Autodesk Fusion 360 part; units mm, degrees
sketch "Sketch1" plane through (0, 0, 0) normal (0, 1, 0) x (1, 0, 0)
  line L0 (0, 0) -> (65, 0)
  line L1 (65, 0) -> (65, 5)
  line L2 (65, 5) -> (80, 5)
  line L3 (80, 5) -> (80, -35)
  line L4 (80, -35) -> (0, -35)
  line L5 (0, -35) -> (-15, -35)
  line L6 (-15, -35) -> (-15, 5)
  line L7 (-15, 5) -> (0, 5)
  line L8 (0, 5) -> (0, 0)
  line L9 (32.5, 0) -> (32.5, -35) construction
  line L10 (32.5, 0) -> (4.5, 0) construction
  line L11 (32.5, 0) -> (60.5, 0) construction
  line L12 (60.5, 0) -> (60.5, -17) construction
  line L13 (56.5, -17) -> (8.5, -17)
  line L14 (4.5, -21) -> (4.5, -35)
  line L15 (60.5, -21) -> (60.5, -35)
  arc A0 (8.5, -17) -> (4.5, -21) centre (8.5, -21) ccw
  arc A1 (60.5, -21) -> (56.5, -17) centre (56.5, -21) ccw
  point P0 (4.5, -17)
  dimension "d1" = 65
  dimension "d2" = 28
  dimension "d3" = 28
  dimension "d4" = 17
  dimension "d5" = 56
  dimension "d6" = 4
  dimension "d7" = 4
extrude "Extrude1" add sketch "Sketch1" along normal blind 50 contours L0 L1 L2 L3 L4 L5 L6 L7 L8 L13 L14 L15 A0 A1
sketch "Sketch2" plane through (0, 0, 35) normal (0, 0, 1) x (1, 0, 0)
  line L0 (-15, 0) -> (4.5, 0)
  line L1 (4.5, 0) -> (4.5, 50)
  line L2 (4.5, 50) -> (-15, 50)
  line L3 (-15, 50) -> (-15, 0)
  line L4 (-15, 25) -> (80, 25) construction
  line L5 (32.5, 0.0866) -> (32.5, 50) construction
  line L6 (32.5, 25) -> (72.5, 25) construction
  line L7 (72.5, 25) -> (72.5, 41.75) construction
  line L8 (72.5, 25) -> (72.5, 8.25) construction
  line L9 (72.5, 41.75) -> (-7.5, 41.75) construction
  line L10 (72.5, 8.25) -> (-7.5, 8.25) construction
  point P0 (-7.5, 41.75)
  point P1 (72.5, 41.75)
  point P2 (72.5, 8.25)
  point P3 (-7.5, 8.25)
  dimension "d10" = 40
  dimension "d11" = 16.75
  dimension "d12" = 16.75
  dimension "d13" = 80
  dimension "d14" = 80
hole "Hole1" at (-7.5, 41.75, 35) at (72.5, 41.75, 35) at (72.5, 8.25, 35) at (-7.5, 8.25, 35) direction (0, 0, -1) diameter 5.5 depth 40 tip angle 118 counterbore diameter 9 counterbore depth 22
sketch "Sketch3" plane through (80, 0, 0) normal (1, 0, 0) x (0, 0, -1)
  line L0 (-35, 0) -> (5, 0)
  line L1 (5, 0) -> (5, 50)
  line L2 (5, 50) -> (-35, 50)
  line L3 (-35, 50) -> (-35, 0)
  line L4 (5, 25) -> (-35, 25) construction
  line L5 (-28.6189, 25) -> (-28.6189, 33) construction
  line L6 (-28.6189, 33) -> (-28.6189, 17) construction
  point P0 (-28.6189, 33)
  point P1 (-28.6189, 17)
hole "Hole2" at (80, 17, 28.6189) at (80, 33, 28.6189) direction (-1, 0, 0) diameter 3.2 depth 40 tip angle 118 counterbore diameter 7 counterbore depth 10
The model under review builds one solid part; all positions refer to its coordinate system, in mm. A direction names the side the tool comes from. Round coordinates to 2 decimals unless told otherwise and drop trailing zeros. Order: outer loops, then holes, each group sorted by start corner. A loop starts at its lowest first (then second) coordinate and runs counter-clockwise, first axis right, second up. Notation, with made-up numbers: (-21, 7) -> (14, 7) arc R20 ccw to (14, 22) -> close; hole circle Ø9 at (-11, 36). An arc over 180 degrees is marked (long way). One line per item, written item: value. Start each with the question number.
Q1. Clearance check with flat-ended pins moving along their axes: pin 1 Ø12 at (x, z) = (8.5, 21.5) entering from +Y; pin 2 Ø8 at (x, y) = (48.5, 25.5) entering from -Z; pin 3 Ø6 at (x, y) = (50, 28) entering from +Z; pin 4 Ø6.5 at (x, y) = (72.5, 8.25) entering from +Z. State where each tip first meets the part, or that it passes through.
Q2. Wall thickness on line 1 (Y direction, x = -7.5, z = 29.5); line 2 (X direction, y = 8, z = 7); line 3 (Z direction, x = 73, y = 17): over which ranges is each line inside the solid? List them lowest first.
Q3. Take a section at D-D (z = 7). Write out the cut boundary in (x, y).
Q4. Machinability: for faces 4 (the face through (70, 34, 27)), 5 (the face through (33, 25, 17)), 6 (the face through (-5, 25, 35)), 7 (the face through (65, 25, -2)), 8 (the face through (68.706, 39.331, 23.846)), which of the approach directions +Z, -Z, +X, -X, +Y, -Y give a long, thin tool a straight path to every point of the face, cutting with its end or side? Answer none if there is none.
Q5. Take a section at A-A (x = 72.5). Write out the cut boundary in (y, z), and give its area (3 significant figures).
Q6. Take a section at C-C (y = 17). Write out the cut boundary in (x, z).
Q7. Take a section at B-B (z = 23.5). Write out the cut boundary in (x, y).
Q8. Mouldability with a two-part tool opening along Y and no side actions: class faces 1 (the face through (32, 50, 15)), 2 (the face through (4.5, 25, 28)), 3 (the face through (-7.6, 44.5, 3.9)) as released by +Y, released by -Y, zero draft, split by the parting line, or undercut.
Reported:
1. pin 1: stops at y = 50
1. pin 2: stops at z = 0
1. pin 3: stops at z = 17
1. pin 4: stops at z = 13
2. line 1: y = 0 to 3.75, 12.75 to 37.25, 46.25 to 50
2. line 2: x = -15 to -10.24, -4.76 to 69.76, 75.24 to 80
2. line 3: z = -5 to 25.12, 32.12 to 35
3. outline: (-15, 0) -> (80, 0) -> (80, 50) -> (-15, 50) -> close; hole circle Ø5.5 at (-7.5, 8.25); hole circle Ø5.5 at (-7.5, 41.75); hole circle Ø5.5 at (72.5, 8.25); hole circle Ø5.5 at (72.5, 41.75)
4. face 4: +X
4. face 5: +Z, +Y, -Y
4. face 6: +Z, +X, -X, +Y, -Y
4. face 7: -Z, +Y, -Y
4. face 8: +Z
5. outline: (0, -5) -> (5.5, -5) -> (5.5, 13) -> (3.75, 13) -> (3.75, 35) -> (0, 35) -> close; (11, -5) -> (39, -5) -> (39, 13) -> (37.25, 13) -> (37.25, 35) -> (12.75, 35) -> (12.75, 13) -> (11, 13) -> close; (44.5, -5) -> (50, -5) -> (50, 35) -> (46.25, 35) -> (46.25, 13) -> (44.5, 13) -> close; hole circle Ø7 at (17, 28.62); hole circle Ø7 at (33, 28.62)
5. area: 1,330 mm2
6. outline: (-15, -5) -> (0, -5) -> (0, 0) -> (65, 0) -> (65, -5) -> (80, -5) -> (80, 25.12) -> (70, 25.12) -> (70, 27.02) -> (60.5, 27.02) -> (60.5, 21) arc R4 cw to (56.5, 17) -> (8.5, 17) arc R4 cw to (4.5, 21) -> (4.5, 35) -> (-15, 35) -> close; (60.5, 30.22) -> (70, 30.22) -> (70, 32.12) -> (80, 32.12) -> (80, 35) -> (60.5, 35) -> close
7. outline: (-15, 0) -> (4.5, 0) -> (4.5, 50) -> (-15, 50) -> close; (60.5, 0) -> (80, 0) -> (80, 50) -> (60.5, 50) -> close; hole circle Ø9 at (-7.5, 8.25); hole circle Ø9 at (-7.5, 41.75); hole circle Ø9 at (72.5, 8.25); hole circle Ø9 at (72.5, 41.75)
8. face 1: released by +Y
8. face 2: zero draft
8. face 3: undercut
